The drawing under review shows one solid part. Ordinate dimensions are in mm from its lowest x, y, z. A direction names the side the tool comes from. Coordinates: 2 decimals unless noted, no trailing zeros. Write each loop counter-clockwise with the first axis right and the second up, starting at its lowest first coordinate (ties: lowest second). Pieces come first, ordered by that corner, then holes.
Q1. Take a section at B-B (y = 38.1). Give the boundary of the cut face in (x, z) (3 decimals).
Q2. Take a section at C-C (x = 16). Give the boundary of the cut face in (y, z) (3 decimals), and give its area (3 significant figures).
Q3. Mouldability with a two-part tool opening along X and no side actions: class the marked faces 1, 2 and 3 as pulls with the +X half, pulls with the -X half, needs draft (parallel to the pull), parting line crosses it, or undercut.
Q4. Take a section at A-A (z = 12.7). Give the boundary of the cut face in (x, y) (3 decimals), and give its area (3 significant figures).
Q5. Insertion check: pin 1 (8 mm diameter, centred on x = 24.5, z = 19, fed in from +Y); pin 2 (12.5 mm diameter, centred on x = 15, y = 30.5, fed in from -Z). Each pin has a flat end and moves straight along its axis. Give the tip position at first contact, or say it passes through.
Q6. Machinability: for the marked faces 4 and 5, which of the approach directions +Z, -Z, +X, -X, +Y, -Y give a long, thin tool a straight path to every point of the face, cutting with its end or side? Answer none if there is none.
Q7. For probe 1 along Y at (x, z) = (30.9, 12.7); probe 2 along X at (y, z) = (10.5, 10) (3 decimals); probe 3 along Z at (x, y) = (16, 7) (3 decimals), list the stretches that pass through material, from the lowest coordinate up.
Q8. Take a section at D-D (y = 21.5). Give the boundary of the cut face in (x, z) (3 decimals).
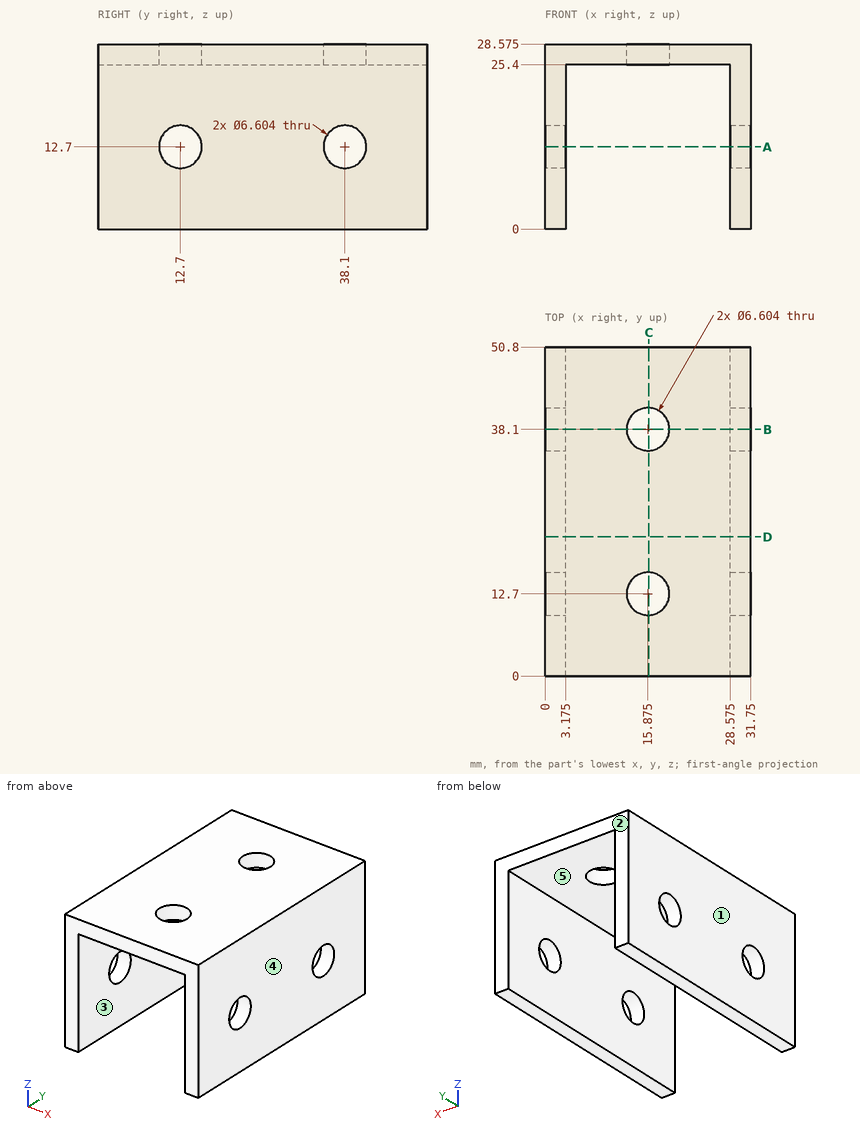
Response:
1. outline: (0, 0) - (3.175, 0) - (3.175, 9.398) - (0, 9.398) - close; (0, 16.002) - (3.175, 16.002) - (3.175, 25.4) - (12.573, 25.4) - (12.573, 28.575) - (0, 28.575) - close; (19.177, 25.4) - (28.575, 25.4) - (28.575, 16.002) - (31.75, 16.002) - (31.75, 28.575) - (19.177, 28.575) - close; (28.575, 0) - (31.75, 0) - (31.75, 9.398) - (28.575, 9.398) - close
2. outline: (0, 25.4) - (9.4, 25.4) - (9.4, 28.575) - (0, 28.575) - close; (16, 25.4) - (34.8, 25.4) - (34.8, 28.575) - (16, 28.575) - close; (41.4, 25.4) - (50.8, 25.4) - (50.8, 28.575) - (41.4, 28.575) - close
2. area: 119 mm2
3. face 1: pulls with the -X half
3. face 2: needs draft
3. face 3: undercut
4. outline: (0, 0) - (3.175, 0) - (3.175, 9.398) - (0, 9.398) - close; (0, 16.002) - (3.175, 16.002) - (3.175, 34.798) - (0, 34.798) - close; (0, 41.402) - (3.175, 41.402) - (3.175, 50.8) - (0, 50.8) - close; (28.575, 0) - (31.75, 0) - (31.75, 9.398) - (28.575, 9.398) - close; (28.575, 16.002) - (31.75, 16.002) - (31.75, 34.798) - (28.575, 34.798) - close; (28.575, 41.402) - (31.75, 41.402) - (31.75, 50.8) - (28.575, 50.8) - close
4. area: 239 mm2
5. pin 1: passes through
5. pin 2: stops at z = 25.4
6. face 4: +Z, -Z, +X, +Y, -Y
6. face 5: -Z, +Y, -Y
7. probe 1: y = 0 to 9.4, 16 to 34.8, 41.4 to 50.8
7. probe 2: x = 0 to 3.175, 28.575 to 31.75
7. probe 3: z = 25.4 to 28.575
8. outline: (0, 0) - (3.175, 0) - (3.175, 25.4) - (28.575, 25.4) - (28.575, 0) - (31.75, 0) - (31.75, 28.575) - (0, 28.575) - close
